from build123d import *

# Parameters (mm, degrees)
BOSS_EXTRUDE1_DEPTH         = 50.8
SKETCH2_R                   = 12.7
CUT_EXTRUDE1_DEPTH          = 44.45
F_1_4_20_TAPPED_HOLE1_D     = 5.1054
F_1_4_20_TAPPED_HOLE1_DEPTH = 6.35
SKETCH5_R                   = 3.3782
CUT_EXTRUDE2_DEPTH          = 8.89
SKETCH6_R                   = 9.525
CUT_EXTRUDE3_DEPTH          = 8.89
FILLET1_RADIUS              = 25.4
FILLET1_LENGTH              = 6.35


with BuildPart() as part:
    # Sketch1 → Boss-Extrude1 (new body)
    with BuildSketch(Plane.XY):
        Polygon((0, 0), (6.35, 0), (6.35, 88.9), (0, 88.9), (0, 63.5), (-31.75, 63.5), (-31.75, 88.9), (-38.1, 88.9), (-38.1, 57.15), (0, 57.15), align=None)
    extrude(amount=BOSS_EXTRUDE1_DEPTH)

    # Sketch2 → Cut-Extrude1 (cut)
    with BuildSketch(Plane.ZY):
        with Locations(Location((25.4, 28.575, 0), (0, 0, 270))):
            Circle(SKETCH2_R)
    extrude(amount=-CUT_EXTRUDE1_DEPTH, mode=Mode.SUBTRACT)

    # 1/4-20 Tapped Hole1
    with Locations(Plane.ZY):
        with Locations((15.875, 79.375), (34.925, 79.375)):
            Hole(F_1_4_20_TAPPED_HOLE1_D / 2, depth=F_1_4_20_TAPPED_HOLE1_DEPTH)

    # Sketch5 → Cut-Extrude2 (cut)
    with BuildSketch(Plane.ZY.offset(38.1)):
        with Locations((15.875, 79.375)):
            Circle(SKETCH5_R)
        with Locations((34.925, 79.375)):
            Circle(SKETCH5_R)
    extrude(amount=-CUT_EXTRUDE2_DEPTH, mode=Mode.SUBTRACT)

    # Sketch6 → Cut-Extrude3 (cut)
    with BuildSketch(Plane(origin=(0, 63.5, 0), x_dir=(1, 0, 0), z_dir=(0, 1, 0))):
        with Locations(Location((-15.875, -25.4, 0), (0, 0, 270))):
            Circle(SKETCH6_R)
    extrude(amount=-CUT_EXTRUDE3_DEPTH, mode=Mode.SUBTRACT)

    # Fillet1: full round fillet: the end face becomes a half cylinder, R = half its width
    fillet1_face = Plane((3.175, 0, 25.4), x_dir=(1, 0, 0), z_dir=(0, -1, 0))  # on the end face: x along it, z out of the body
    fillet1_slab = fillet1_face.offset(-FILLET1_RADIUS / 2) * Box(FILLET1_LENGTH, 2 * FILLET1_RADIUS, FILLET1_RADIUS, mode=Mode.PRIVATE)  # the body's end, R deep
    fillet1_round = Plane((3.175, 25.4, 25.4), x_dir=(0, -1, 0), z_dir=(1, 0, 0)) * Cylinder(FILLET1_RADIUS, FILLET1_LENGTH, mode=Mode.PRIVATE)  # its axis R under the face
    add(fillet1_slab - fillet1_round, mode=Mode.SUBTRACT)


solid = part.part
Could you check a few things on this model? Use its own coordinates, in mm. A direction names the side the tool comes from. Give positions to 0.01 mm unless a question says otherwise; leave off trailing zeros. Order: outer loops, then holes, each group sorted by start corner. A loop starts at its lowest first (then second) coordinate and runs counter-clockwise, first axis right, second up.
1. Suppose I cut it at C-C (x = -17.5). List the corners of the cut face in (y, z) for me.
2. We'd pull the mould along Z, two halves only. Please class faces 4 (the cylindrical face through (3.219, 0.006, 25.959)), 5 (the flat face through (-13, 62, 0)), 6 (the flat face through (0, 42, 25)), 7 (the cylindrical face through (3.219, 76.883, 35.478)): pulls with the +Z half, pulls with the -Z half, needs draft (parallel to the pull), parting line crosses it, or undercut.
3. For faces 1 (the cylindrical face through (-34.969, 76.378, 17.434)), 2 (the flat face through (0, 76, 25)), 3 (the flat face through (-24, 57.15, 19)), which set-ups out of +Z, -Z, +X, -X, +Y, -Y let a thin tool reach every point of the face, with its end or its side?
4. Suppose I cut it at A-A (z = 25.4). List the corners of the cut face in (x, y) for me (3 decimals).
5. Suppose I cut it at B-B (y = 32). List the corners of the cut face in (x, z) for me.
6. Will these pins go through, and if not, where does the flat tip stop? P1, Ø25, axis at x = -15.875, z = 25.4, coming from the +Y side; P2, Ø12, axis at y = 44.5, z = 20.5, coming from the -X side.
7. I need wall thicknesses on L1, parallel to X at y = 71, z = 11.5; L2, parallel to Y at x = -29, z = 4.5; L3, parallel to X at y = 47, z = 41.5. Which ranges of each line are inside material? Lowest first, please.
8. Suppose I cut it at D-D (x = 2). List the corners of the cut face in (y, z) for me (3 decimals), plus the area to 3 significant figures.
Solved:
1. outline: (57.15, 0) - (63.5, 0) - (63.5, 16.01) - (57.15, 16.01) - close; (57.15, 34.79) - (63.5, 34.79) - (63.5, 50.8) - (57.15, 50.8) - close
2. face 4: parting line crosses it
2. face 5: pulls with the -Z half
2. face 6: needs draft
2. face 7: undercut
3. face 1: -X
3. face 2: +Z, -Z, +Y
3. face 3: +Z, -Z, -X, -Y
4. outline: (-38.1, 57.15) - (-25.4, 57.15) - (-25.4, 63.5) - (-31.75, 63.5) - (-31.75, 88.9) - (-38.1, 88.9) - close; (-6.35, 57.15) - (0, 57.15) - (0, 41.275) - (6.35, 41.275) - (6.35, 88.9) - (0, 88.9) - (0, 63.5) - (-6.35, 63.5) - close; (0, 0) - (6.35, 0) - (6.35, 15.875) - (0, 15.875) - close
5. outline: (0, 0) - (6.35, 0) - (6.35, 13.17) - (0, 13.17) - close; (0, 37.63) - (6.35, 37.63) - (6.35, 50.8) - (0, 50.8) - close
6. P1: stops at y = 63.5
6. P2: stops at x = 0
7. L1: x = -38.1 to -31.75, 0 to 6.35
7. L2: y = 57.15 to 63.5
7. L3: x = 0 to 6.35
8. outline: (25.4, 0) - (88.9, 0) - (88.9, 50.8) - (25.4, 50.8) arc R25.4 ccw to start; hole circle Ø25.4 at (28.575, 25.4); hole circle Ø5.105 at (79.375, 15.875); hole circle Ø5.105 at (79.375, 34.925)
8. area: 3,690 mm2
